```python
from build123d import *

# Parameters (mm, degrees)
F0_W     = 76
F0_H     = 147
F0_W_2   = 72
F0_H_2   = 143
F1_DEPTH = 2
F2_W     = 76
F2_H     = 147
F2_W_2   = 72
F2_H_2   = 143
F3_DEPTH = 5
F4_R     = 2
F5_W     = 15
F5_H     = 2.5
F6_DEPTH = 5
F7_W     = 30
F7_H     = 2.5
F8_DEPTH = 25


with BuildPart() as f1:
    # F0 (on Top) → F1 (new body)
    with BuildSketch(Plane.XY):
        with Locations((36, 71.5)):
            Rectangle(F0_W, F0_H)
        with Locations((36, 71.5)):
            Rectangle(F0_W_2, F0_H_2, mode=Mode.SUBTRACT)
        with Locations((36, 71.5)):
            Rectangle(F0_W_2, F0_H_2)
    extrude(amount=F1_DEPTH)

    # F2 (on face) → F3 (join)
    with BuildSketch(Plane.XY.offset(2)):
        with Locations((36, 71.5)):
            Rectangle(F2_W, F2_H)
        with Locations((36, 71.5)):
            Rectangle(F2_W_2, F2_H_2, mode=Mode.SUBTRACT)
    extrude(amount=F3_DEPTH)

    # F4
    f4_edges = [f1.edges().sort_by_distance(p)[0] for p in [
        (36, 143, 2),
        (72, 71.5, 2),
        (36, 0, 2),
        (0, 71.5, 2),
        (36, 145, 0),
        (-2, 71.5, 0),
        (36, -2, 0),
        (74, 71.5, 0),
        (74, -2, 3.5),
        (-2, -2, 3.5),
        (-2, 145, 3.5),
        (74, 145, 3.5),
        (72, 0, 4.5),
        (0, 0, 4.5),
        (0, 143, 4.5),
        (72, 143, 4.5),
    ]]
    fillet(f4_edges, radius=F4_R)

    # F5 (on face) → F6 (cut)
    with BuildSketch(Plane.YZ.offset(74)):
        with Locations((100.5, 4.25)):
            Rectangle(F5_W, F5_H)
    extrude(amount=-F6_DEPTH, mode=Mode.SUBTRACT)

    # F7 (on face) → F8 (cut)
    with BuildSketch(Plane(origin=(-2, 0, 0), x_dir=(0, -1, 0), z_dir=(-1, 0, 0))):
        with Locations((-108, 4.25)):
            Rectangle(F7_W, F7_H)
    extrude(amount=-F8_DEPTH, mode=Mode.SUBTRACT)


solid = f1.part
```
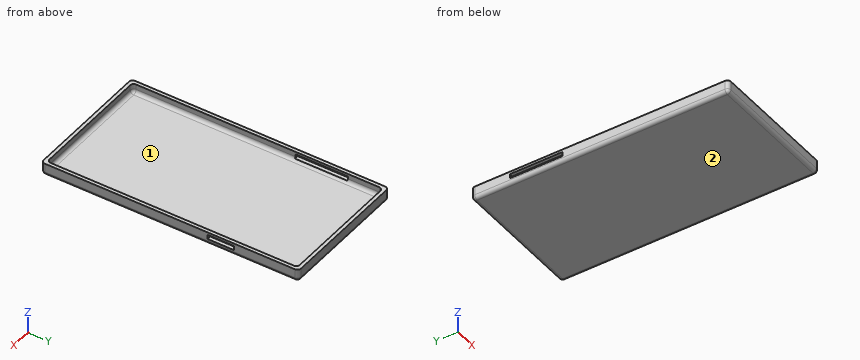
Can you work these out from the model? Positions are in its coordinate system, mm. Face numbers are marked on the shaded views. Round coordinates to 2 decimals unless told otherwise and drop trailing zeros. Loops run counter-clockwise (first coordinate to the right, second up) from the corner with the lowest first, then second, coordinate; pieces in that order, holes last. Notation, with made-up numbers: (24, -20) -> (79, -20) arc R14 ccw to (79, -16) -> close; hole circle Ø4 at (64.25, -8). An arc over 180 degrees is marked (long way). One line per item, written item: value. Start each with the question number.
1. If we section it at A-A, the plane x = 9: Write out the boundary of the cut face in (y, z), then the cut area to 3 significant figures.
2. If we mould it in two halves opening along Y, with no side actions, what happens to the marked faces 1 and 2? For each: pulls with the +Y half, pulls with the -Y half, needs draft (parallel to the pull), parting line crosses it, or undercut.
3. If we section it at B-B, the plane y = 30: Write out the boundary of the cut face in (x, z).
4. If I drill on probe 1 along Y at (x, z) = (5, 3.75); probe 2 along X at (y, z) = (23, 4); probe 3 along Y at (x, z) = (68, 3.5), over which ranges is the centre line in solid material (lowest first)?
5. For pin 1 (1.8 mm diameter, centred on x = -1, z = 4.5, fed in from -Y); pin 2 (4 mm diameter, centred on x = 32, y = 103.5, fed in from +Z); pin 3 (0.6 mm diameter, centred on x = -0.5, y = 109.5, fed in from -Z); pin 4 (2.5 mm diameter, centred on x = -0.5, z = 4.5, fed in from +Y), each with a flat end and sliding along its axis, tell me the tip position at first contact or that it passes through.
Calculated:
1. outline: (-2, 2) arc R2 ccw to (0, 0) -> (143, 0) arc R2 ccw to (145, 2) -> (145, 7) -> (143, 7) -> (143, 4) arc R2 cw to (141, 2) -> (2, 2) arc R2 cw to (0, 4) -> (0, 7) -> (-2, 7) -> close
1. area: 314 mm²
2. face 1: undercut
2. face 2: needs draft
3. outline: (-2, 2) arc R2 ccw to (0, 0) -> (72, 0) arc R2 ccw to (74, 2) -> (74, 7) -> (72, 7) -> (72, 4) arc R2 cw to (70, 2) -> (2, 2) arc R2 cw to (0, 4) -> (0, 7) -> (-2, 7) -> close
4. probe 1: y = -2 to 0.02, 142.98 to 145
4. probe 2: x = -2 to 0, 72 to 74
4. probe 3: y = -2 to 0.06, 142.94 to 145
5. pin 1: stops at y = -2
5. pin 2: stops at z = 2
5. pin 3: stops at z = 0.01
5. pin 4: stops at y = 145
